Can you work these out from the model? Positions are in its coordinate system, mm. Face numbers are marked on the shaded views. Give positions to 0.01 mm unless a question says otherwise; leave off trailing zeros. Order: outer loops, then holes, each group sorted by start corner. A loop starts at its lowest first (then second) coordinate and runs counter-clockwise, first axis right, second up. Notation, with made-up numbers: (16, 73) - (68, 73) arc R16 cw to (68, 88) - close; hole circle Ø5 at (9, 0). An arc over 180 degrees is marked (long way). Return JSON: item names as keys, results as strings.
```python
from build123d import *

# Parameters (mm, degrees)
F0_W     = 150
F0_H     = 150
F1_DEPTH = 150.000006
F2_R     = 20
F4_D     = 5


with BuildPart() as f1:
    # F0 (on Top) → F1 (new body)
    with BuildSketch(Plane.XY):
        with Locations((0, 10.636854)):
            Rectangle(F0_W, F0_H)
    extrude(amount=-F1_DEPTH)

    # F2
    f2_edges = [f1.edges().sort_by_distance(p)[0] for p in [
        (-75, 85.636854, -75.000003),
        (-75, -64.363146, -75.000003),
        (-75, 10.636854, 0),
        (-75, 10.636854, -150.000006),
        (75, -64.363146, -75.000003),
        (75, 85.636854, -75.000003),
        (75, 10.636854, 0),
        (75, 10.636854, -150.000006),
    ]]
    fillet(f2_edges, radius=F2_R)

    # F4 (through all)
    with Locations(Plane.XY):
        with Locations((7.5, 76.136854), (-7.569213, 76.206067)):
            Hole(F4_D / 2)


solid = f1.part
```
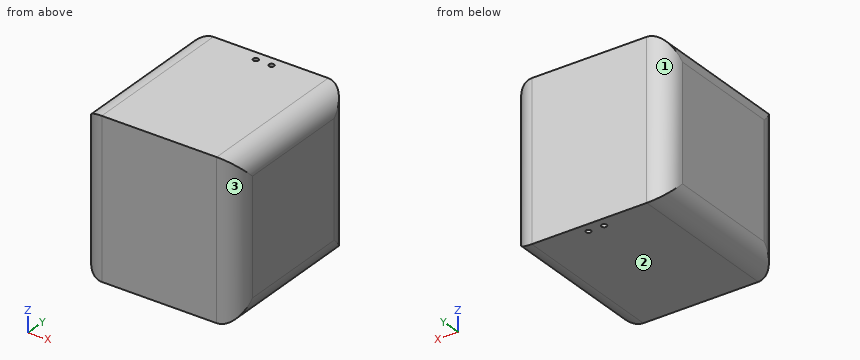
1. If I drill on L1, parallel to Y at x = 7.5, z = -65; L2, parallel to Z at x = -67, y = -42.5; L3, parallel to X at y = -50.5, z = -131, over which ranges is the centre line in solid material (lowest first)? Write a range as [from, to].
Checks:
{"L1": "[-64.36, 73.64], [78.64, 85.64]", "L2": "[-146, -4]", "L3": "[-74.04, 74.04]"}
2. Suppose I cut it at B-B (z = -15). List the corners of the cut face in (x, y) for me, plus the area to 3 significant figures.
Checks:
{"outline": "(-74.36, -49.36) arc R20 ccw to (-55, -64.36) - (55, -64.36) arc R20 ccw to (74.36, -49.36) - (74.36, 70.64) arc R20 ccw to (55, 85.64) - (-55, 85.64) arc R20 ccw to (-74.36, 70.64) - close; hole circle Ø5 at (-7.57, 76.21); hole circle Ø5 at (7.5, 76.14)", "area": "22,000 mm^2"}
3. Thinking about a two-plate mould opening in X: for the marked faces 1, 2 and 3, which applies, +X half, -X half, draft (parallel to the pull), parting line (faces both ways), or undercut?
Checks:
{"face 1": "-X half", "face 2": "draft", "face 3": "+X half"}
4. Suppose I cut it at D-D (z = -47.5). List the corners of the cut face in (x, y) for me.
Checks:
{"outline": "(-75, -44.36) arc R20 ccw to (-55, -64.36) - (55, -64.36) arc R20 ccw to (75, -44.36) - (75, 65.64) arc R20 ccw to (55, 85.64) - (-55, 85.64) arc R20 ccw to (-75, 65.64) - close; hole circle Ø5 at (-7.57, 76.21); hole circle Ø5 at (7.5, 76.14)"}
5. Suppose I cut it at A-A (x = 7.5). List the corners of the cut face in (y, z) for me.
Checks:
{"outline": "(-64.36, -150) - (73.64, -150) - (73.64, 0) - (-64.36, 0) - close; (78.64, -150) - (85.64, -150) - (85.64, 0) - (78.64, 0) - close"}
6. Suppose I cut it at C-C (y = 3). List the corners of the cut face in (x, z) for me.
Checks:
{"outline": "(-75, -130) arc R20 ccw to (-55, -150) - (55, -150) arc R20 ccw to (75, -130) - (75, -20) arc R20 ccw to (55, 0) - (-55, 0) arc R20 ccw to (-75, -20) - close"}
7. For pin 1 Ø4 at (x, y) = (7.5, 76.14) entering from -Z, with a flat end and sliding along its axis, tell me the tip position at first contact or that it passes through.
Checks:
{"pin 1": "through"}
